Geometry check sheet. Reference: the model listing, model coordinates, mm. A direction names the side the tool comes from. Coordinates: 2 decimals unless noted, no trailing zeros. Order: outer loops, then holes, each group sorted by start corner. A loop starts at its lowest first (then second) coordinate and runs counter-clockwise, first axis right, second up. Notation, with made-up numbers: M 13.5,-30 L 68.5,-30 A21 cw 68.5,4 Z; hole C -30,-24.75 d2. An arc over 180 degrees is marked long. One line per item, written item: value. Start each with the question number.
1) Draft check along Y on faces 1 (the flat face through (0, -7, 0)), 2 (the flat face through (0, 8.25, 10)), 3 (the flat face through (0, 2, 5)). Enter one of: pulls with the +Y half, pulls with the -Y half, needs draft (parallel to the pull), parting line crosses it, or undercut.
2) Sectioned sample at D-D, the plane x = 6. Enter the section's corners in (y, z), then the cut area to 4 significant figures.
3) Thickness scan on L1, parallel to Y at x = -10, z = 11.75; L2, parallel to Z at x = -14.5, y = 2.75; L3, parallel to Y at x = 11, z = 6. Record the ranges inside material, lowest first. Write a range as from..to.
4) Sectioned sample at B-B, the plane x = -10. Enter the section's corners in (y, z).
5) Go/stop test with flat-tipped pins: P1, Ø2, axis at x = 0, y = 0, coming from the -Z side; P2, Ø4, axis at x = -10, y = 0, coming from the -Z side. Record where each tip stops, or that it passes through.
6) Sectioned sample at A-A, the plane y = 0.75. Enter the section's corners in (x, z), then the cut area to 3 significant figures.
7) Access from +Z, -Z, +X, -X, +Y, -Y to the whole of each face (thin tool, end or side, straight path). Record for faces 4 (the flat face through (0, -5.25, 2)), 5 (the cylindrical face through (-0.27, -1.22, 12.6)).
8) Sectioned sample at C-C, the plane z = 13. Enter the section's corners in (x, y), then the cut area to 3 significant figures.
```python
from build123d import *

# Parameters (mm, degrees)
F0_W     = 40
F0_H     = 3
F0_H_2   = 10.5
F1_DEPTH = 20
F2_DEPTH = 5
F3_R     = 1.25
F4_DEPTH = 20.001
F5_DEPTH = 20.001


with BuildPart() as f1:
    # F0 (on Top) → F1 (new body)
    with BuildSketch(Plane.XY):
        with Locations((0, 6.75)):
            Rectangle(F0_W, F0_H)
        Rectangle(F0_W, F0_H_2)
        with Locations((0, -6.75)):
            Rectangle(F0_W, F0_H)
    extrude(amount=F1_DEPTH)

    # F0 (on Top) → F2 (cut)
    with BuildSketch(Plane.XY):
        Rectangle(F0_W, F0_H_2)
    extrude(amount=F2_DEPTH, mode=Mode.SUBTRACT)

    # F3 (on face) → F4 (cut, through all)
    with BuildSketch(Plane.XY.offset(20)):
        Circle(F3_R)
    extrude(amount=-F4_DEPTH, mode=Mode.SUBTRACT)

    # F3 (on face) → F5 (cut, through all)
    with BuildSketch(Plane.XY.offset(20)):
        with Locations((10, 0)):
            Circle(F3_R)
        Circle(F3_R)
        with Locations((-10, 0)):
            Circle(F3_R)
    extrude(amount=-F5_DEPTH, mode=Mode.SUBTRACT)


solid = f1.part
```
Final values:
1. face 1: needs draft
1. face 2: pulls with the +Y half
1. face 3: undercut
2. outline: M -8.25,0 L -5.25,0 L -5.25,5 L 5.25,5 L 5.25,0 L 8.25,0 L 8.25,20 L -8.25,20 Z
2. area: 277.5 mm^2
3. L1: y = -8.25..-1.25, 1.25..8.25
3. L2: z = 5..20
3. L3: y = -8.25..-0.75, 0.75..8.25
4. outline: M -8.25,0 L -5.25,0 L -5.25,5 L -1.25,5 L -1.25,20 L -8.25,20 Z; M 1.25,5 L 5.25,5 L 5.25,0 L 8.25,0 L 8.25,20 L 1.25,20 Z
5. P1: passes through
5. P2: stops at z = 5
6. outline: M -20,5 L -11,5 L -11,20 L -20,20 Z; M -9,5 L -1,5 L -1,20 L -9,20 Z; M 1,5 L 9,5 L 9,20 L 1,20 Z; M 11,5 L 20,5 L 20,20 L 11,20 Z
6. area: 510 mm^2
7. face 4: -Z, +X, -X
7. face 5: +Z, -Z
8. outline: M -20,-8.25 L 20,-8.25 L 20,8.25 L -20,8.25 Z; hole C -10,0 d2.5; hole C 0,0 d2.5; hole C 10,0 d2.5
8. area: 645 mm^2
